Check sheet for the modelled part. Datum: model origin and axes. Units: mm. A direction names the side the tool comes from. Coordinates: 2 decimals unless noted, no trailing zeros. Write each loop counter-clockwise with the first axis right and the second up, starting at its lowest first coordinate (ties: lowest second). Pieces come first, ordered by that corner, then holes. Notation, with made-up numbers: M 37.5,71.25 L 47.5,71.25 A32 cw 47.5,106.25 Z; hole C -31.75,-37.5 d3. An arc over 180 degrees is marked long. Answer as CSV lines item,"result".
from build123d import *

# Parameters (mm, degrees)
SKETCH1_R           = 22.57
BOSS_EXTRUDE1_DEPTH = 5
BOSS_EXTRUDE2_DEPTH = 5
CUT_EXTRUDE2_DEPTH  = 5
SKETCH5_R           = 1.5
CUT_EXTRUDE3_DEPTH  = 5
BOSS_EXTRUDE3_DEPTH = 47.62
CUT_EXTRUDE5_DEPTH  = 47.62


with BuildPart() as part:
    # Sketch1 → Boss-Extrude1 (new body)
    with BuildSketch(Plane(origin=(0, 0, 0), x_dir=(0, 0, -1), z_dir=(1, 0, 0))):
        Circle(SKETCH1_R)
    extrude(amount=BOSS_EXTRUDE1_DEPTH)

    # Sketch3 → Boss-Extrude2 (add)
    with BuildSketch(Plane(origin=(5, 0, 0), x_dir=(0, 0, -1), z_dir=(1, 0, 0))):
        Polygon((21.833735154, 5.717771349), (14.930960802, 30.701130063), (-28.574903185, 18.68068215), (-21.833735154, -5.717771349), align=None)
    extrude(amount=-BOSS_EXTRUDE2_DEPTH)

    # Sketch4 → Cut-Extrude2 (cut)
    with BuildSketch(Plane.ZY):
        Polygon((4.470755169, -4.540778658), (6.167807255, 1.601398221), (1.697052086, 6.142176879), (-4.470755169, 4.540778658), (-6.167807255, -1.601398221), (-1.697052086, -6.142176879), align=None)
    extrude(amount=-CUT_EXTRUDE2_DEPTH, mode=Mode.SUBTRACT)

    # Sketch5 → Cut-Extrude3 (cut)
    with BuildSketch(Plane(origin=(5, 0, 0), x_dir=(0, 0, -1), z_dir=(1, 0, 0))):
        with Locations((0.669304585, -13.687213536)):
            Circle(SKETCH5_R)
        with Locations((6.452618137, -12.089313553)):
            Circle(SKETCH5_R)
    extrude(amount=-CUT_EXTRUDE3_DEPTH, mode=Mode.SUBTRACT)

    # Sketch6 → Boss-Extrude3 (add)
    with BuildSketch(Plane(origin=(5, 0, 0), x_dir=(0, 0, -1), z_dir=(1, 0, 0))):
        Polygon((10.64416617, 27.44177556), (-23.222841897, 18.084494285), (-22.406311475, 15.129208279), (11.460696592, 24.486489554), align=None)
    extrude(amount=BOSS_EXTRUDE3_DEPTH)

    # Sketch7 → Cut-Extrude5 (cut)
    with BuildSketch(Plane(origin=(52.62, 0, 0), x_dir=(0, 0, -1), z_dir=(1, 0, 0))):
        Polygon((11.460696592, 24.486489554), (10.64416617, 27.44177556), (-23.222841897, 18.084494285), (-22.406311475, 15.129208279), align=None)
        Polygon((11.399186479, 24.521368001), (10.609287723, 27.380265447), (-23.161331784, 18.049615839), (-22.371433028, 15.190718392), align=None, mode=Mode.SUBTRACT)
    extrude(amount=-CUT_EXTRUDE5_DEPTH, mode=Mode.SUBTRACT)


solid = part.part
1) Mould release check, pull along Y, two halves, no side actions. Record for faces 1 (the face through (0, 10, 3)), 2 (the face through (2.465, -5.353, 1.344)), 3 (the face through (2.54, 18.33, -18.35)): pulls with the +Y half, pulls with the -Y half, needs draft (parallel to the pull), parting line crosses it, or undercut.
Answer key:
face 1,"needs draft"
face 2,"undercut"
face 3,"pulls with the +Y half"
2) Section check B-B, the plane y = 0. Record the boundary of the cut face in (x, z).
Answer key:
outline,"M 0,-22.57 L 5,-22.57 L 5,-5.73 L 0,-5.73 Z; M 0,5.73 L 5,5.73 L 5,23.41 L 0,23.41 Z"
3) Section check D-D, the plane z = 9. Record the boundary of the cut face in (x, y).
Answer key:
outline,"M 0,-20.7 L 5,-20.7 L 5,18.89 L 52.62,18.89 L 52.62,21.96 L 5,21.96 L 5,24.09 L 0,24.09 Z"
4) Thickness scan on line 1 along X through (y, z) = (-18.5, 5.5); line 2 along Y through (x, z) = (48, -10.5); line 3 along Y through (x, z) = (22, -1.5). Record the ranges inside material, lowest first.
Answer key:
line 1,"x = 0 to 5"
line 2,"y = 24.27 to 27.35"
line 3,"y = 21.79 to 24.86"
5) Section check C-C, the plane x = 11. Record the boundary of the cut face in (y, z), plus the area to 3 significant figures.
Answer key:
outline,"M 15.19,22.37 L 24.52,-11.4 L 27.38,-10.61 L 18.05,23.16 Z"
area,"104 mm2"
6) Tool access check on faces 4 (the face through (29.14, 16.64, 22.77)), 5 (the face through (29.14, 19.79, 5.72)), 6 (the face through (2.46, -1.51, 5.31)). Record the directions out of +Z, -Z, +X, -X, +Y, -Y that give a thin tool (end or side, any length) a straight path to the whole face; none if there is none.
Answer key:
face 4,"+Z, +X, -Y"
face 5,"-Z, +X, -Y"
face 6,"+X, -X"
7) Section check A-A, the plane z = 0. Record the boundary of the cut face in (x, y).
Answer key:
outline,"M 0,-22.57 L 5,-22.57 L 5,-15.03 L 0,-15.03 Z; M 0,-12.34 L 5,-12.34 L 5,-5.7 L 0,-5.7 Z; M 0,5.7 L 5,5.7 L 5,21.37 L 52.62,21.37 L 52.62,24.45 L 5,24.45 L 5,26.58 L 0,26.58 Z"
8) Depth check by flat-ended pin: P1, Ø5, axis at x = 19, z = 10.5, coming from the -Y side; P2, Ø5, axis at y = -17, z = 14, coming from the +X side; P3, Ø1.5, axis at x = 10.5, z = 2, coming from the -Y side; P4, Ø1.8, axis at y = -13.69, z = -0.67, coming from the -X side. Enter the tip coordinate at first touch or a pass-through.
Answer key:
P1,"stops at y = 17.78"
P2,"stops at x = 5"
P3,"stops at y = 20.61"
P4,"passes through"
